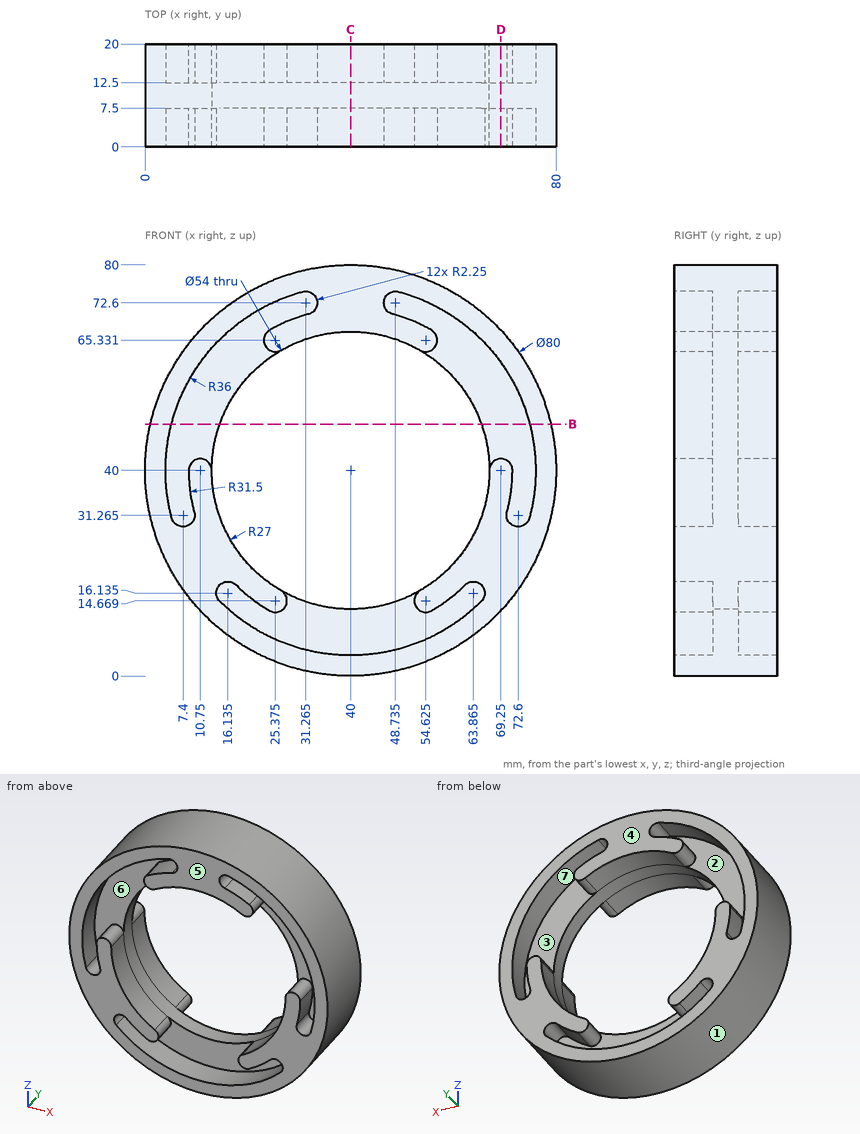
For this review, use the dimensioned drawing (mm, ordinates from the lowest corner) and the shaded views. A direction names the side the tool comes from. Coordinates: 2 decimals unless noted, no trailing zeros. Write each loop counter-clockwise with the first axis right and the second up, starting at its lowest first coordinate (ties: lowest second). Pieces come first, ordered by that corner, then holes. Notation, with made-up numbers: (66.25, 42.5) - (88.25, 42.5) arc R17 cw to (88.25, 57.5) - close; hole circle Ø6 at (41, 59). An arc over 180 degrees is marked (long way). Answer as a JSON object with one key per item and string values. Group by question number.
1. Add section B-B (z = 49). Give the boundary of the cut face in (x, y).
2. Machinability: for the marked faces 5, 6 and 7, which of the approach directions +Z, -Z, +X, -X, +Y, -Y give a long, thin tool a straight path to every point of the face, cutting with its end or side? Answer none if there is none.
3. Mouldability with a two-part tool opening along Z and no side actions: class the marked faces 1, 2, 3 and 4 as pulls with the +Z half, pulls with the -Z half, needs draft (parallel to the pull), parting line crosses it, or undercut.
4. Add section C-C (x = 40). Give the boundary of the cut face in (y, z), plus the area to 3 significant figures.
5. To check wall thickness, follow probe 1 along X at (y, z) = (15.5, 40); probe 2 along X at (y, z) = (11.1, 40); probe 3 along X at (y, z) = (3.5, 14) (1 decimal). State the ranges of each line that lie inside material, in increasing order.
6. Clearance check with flat-ended pins moving along their axes: pin 1 Ø10 at (y, z) = (10.5, 25.5) entering from -X; pin 2 Ø4 at (x, y) = (31.5, 8.5) entering from +Z; pin 3 Ø9 at (x, z) = (21.5, 55) entering from +Y. State where each tip first meets the part, or that it passes through.
7. Add section D-D (x = 69.25). Give the boundary of the cut face in (y, z), plus the area to 3 significant figures.
Findings:
{
 "1": {"outline": "(1.03, 0) - (5.14, 0) - (5.14, 7.5) - (14.54, 7.5) - (14.54, 12.5) - (5.14, 12.5) - (5.14, 20) - (1.03, 20) - close; (65.46, 7.5) - (74.86, 7.5) - (74.86, 0) - (78.97, 0) - (78.97, 20) - (74.86, 20) - (74.86, 12.5) - (65.46, 12.5) - close"},
 "2": {"face 5": "+Z, -Z, +X, -X, -Y", "face 6": "-Y", "face 7": "+Y"},
 "3": {"face 1": "parting line crosses it", "face 2": "undercut", "face 3": "undercut", "face 4": "needs draft"},
 "4": {"outline": "(0, 0) - (20, 0) - (20, 4) - (12.5, 4) - (12.5, 13) - (7.5, 13) - (7.5, 4) - (0, 4) - close; (0, 67) - (20, 67) - (20, 80) - (0, 80) - close", "area": "385 mm²"},
 "5": {"probe 1": "0 to 4, 8.5 to 13, 67 to 71.5, 76 to 80", "probe 2": "0 to 13, 67 to 80", "probe 3": "9.6 to 15.1, 22.2 to 27.5, 52.5 to 57.8, 64.9 to 70.4"},
 "6": {"pin 1": "x = 1.14", "pin 2": "z = 79.47", "pin 3": "y = 12.5"},
 "7": {"outline": "(0, 12.72) - (20, 12.72) - (20, 42.25) - (12.5, 42.25) - (12.5, 60.99) - (20, 60.99) - (20, 67.28) - (0, 67.28) - (0, 60.99) - (7.5, 60.99) - (7.5, 42.25) - (0, 42.25) - close", "area": "810 mm²"}
}
